Can you work these out from the model? Positions are in its coordinate system, mm. A direction names the side the tool comes from. Round coordinates to 2 decimals unless told otherwise and drop trailing zeros. Loops run counter-clockwise (first coordinate to the right, second up) from the corner with the lowest first, then second, coordinate; pieces in that order, holes last. Notation, with made-up numbers: (40, 41.5) -> (66, 41.5) arc R32 cw to (66, 76.5) -> close; hole circle Ø4 at (75.25, 85.25). An arc over 180 degrees is marked (long way). Use a Markdown table: item, result.
from build123d import *

# Parameters (mm, degrees)
SALIENTE_EXTRUIR1_DEPTH = 28
VACIADO2_START          = 6
VACIADO2_OUTLINE_W      = 16
VACIADO2_OUTLINE_H      = 23
VACIADO2_DEPTH          = 21
CORTAR_EXTRUIR1_REACH   = 46.204
CROQUIS2_W              = 6.4
CROQUIS2_H              = 10
CORTAR_EXTRUIR2_REACH   = 46.204
CROQUIS4_W              = 6.4
CROQUIS4_H              = 10


# Read off the part's stored shape, not the designer's step: Vaciado2
with BuildPart() as part:
    # Croquis1 → Saliente-Extruir1 (new body)
    with BuildSketch(Plane(origin=(0, 0, 0), x_dir=(0, 0, -1), z_dir=(1, 0, 0))):
        Polygon((0, 0), (27, 0), (27, 27), (21, 27), (0, 6), align=None)
    extrude(amount=SALIENTE_EXTRUIR1_DEPTH)

    # Vaciado2 outline → Vaciado2 (cut)
    with BuildSketch(Plane(origin=(0, 0, 0), x_dir=(1, 0, 0), z_dir=(0, 1, 0)).offset(VACIADO2_START)):
        with Locations((14, 9.5)):
            Rectangle(VACIADO2_OUTLINE_W, VACIADO2_OUTLINE_H)
    extrude(amount=VACIADO2_DEPTH, mode=Mode.SUBTRACT)

    # Croquis2 → Cortar-Extruir1 (cut, up to next)
    with BuildSketch(Plane.XY.offset(-21), mode=Mode.PRIVATE) as cortar_extruir1_sk1:
        with Locations((14, 15)):
            Rectangle(CROQUIS2_W, CROQUIS2_H)
    cortar_extruir1_tool1 = extrude(cortar_extruir1_sk1.sketch, amount=-CORTAR_EXTRUIR1_REACH, mode=Mode.PRIVATE) & part.part
    add(cortar_extruir1_tool1.solids().sort_by_distance((14, 15, -21))[0], mode=Mode.SUBTRACT)

    # Croquis4 → Cortar-Extruir2 (cut, up to next)
    with BuildSketch(Plane(origin=(0, 6, 0), x_dir=(1, 0, 0), z_dir=(0, 1, 0)), mode=Mode.PRIVATE) as cortar_extruir2_sk1:
        with Locations((14, 12)):
            Rectangle(CROQUIS4_W, CROQUIS4_H)
    cortar_extruir2_tool1 = extrude(cortar_extruir2_sk1.sketch, amount=-CORTAR_EXTRUIR2_REACH, mode=Mode.PRIVATE) & part.part
    add(cortar_extruir2_tool1.solids().sort_by_distance((14, 6, -12))[0], mode=Mode.SUBTRACT)


solid = part.part
1. Which directions (+Z, -Z, +X, -X, +Y, -Y) give clear straight access to the entire face, cutting with the end or side of a thin tool? Please do faces 1 (the flat face through (10, 6, -11)), 2 (the flat face through (17.2, 3, -12)), 3 (the flat face through (14, 10, -24)).
Answer sheet:
| item | result |
|---|---|
| face 1 | +Z, +Y |
| face 2 | +Y, -Y |
| face 3 | +Z, -Z |
2. If we mould it in two halves opening along Z, with no side actions, what happens to faces 4 (the flat face through (14, 3, 0)), 5 (the flat face through (22, 12, -15)), 6 (the flat face through (14, 3, -7))? For each: +Z half, -Z half, draft (parallel to the pull), parting line (faces both ways), or undercut.
Answer sheet:
| item | result |
|---|---|
| face 4 | +Z half |
| face 5 | draft |
| face 6 | undercut |
3. I want a section at C-C (z = -24). Please give me the cut outline in (x, y).
Answer sheet:
| item | result |
|---|---|
| outline | (0, 0) -> (28, 0) -> (28, 27) -> (0, 27) -> close; hole (10.8, 10) -> (17.2, 10) -> (17.2, 20) -> (10.8, 20) -> close |
4. I want a section at D-D (y = 5.5). Please give me the cut outline in (x, z).
Answer sheet:
| item | result |
|---|---|
| outline | (0, -27) -> (28, -27) -> (28, 0) -> (0, 0) -> close; hole (10.8, -17) -> (17.2, -17) -> (17.2, -7) -> (10.8, -7) -> close |
5. Will these pins go through, and if not, where does the flat tip stop? pin 1 Ø1 at (y, z) = (15.5, -8) entering from -X; pin 2 Ø12 at (x, z) = (22, -9.5) entering from +Y; pin 3 Ø8 at (x, z) = (9.5, -14) entering from +Y; pin 4 Ø1.5 at (x, y) = (9, 10) entering from +Z.
Answer sheet:
| item | result |
|---|---|
| pin 1 | passes through |
| pin 2 | stops at y = 21.5 |
| pin 3 | stops at y = 21.94 |
| pin 4 | stops at z = -21 |
6. I want a section at B-B (x = 16). Please give me the cut outline in (y, z).
Answer sheet:
| item | result |
|---|---|
| outline | (0, -27) -> (10, -27) -> (10, -21) -> (6, -21) -> (6, -17) -> (0, -17) -> close; (0, -7) -> (6, -7) -> (6, 0) -> (0, 0) -> close; (20, -27) -> (27, -27) -> (27, -21) -> (20, -21) -> close |
7. I want a section at A-A (y = 19.25). Please give me the cut outline in (x, z), plus the area to 3 significant figures.
Answer sheet:
| item | result |
|---|---|
| outline | (0, -27) -> (10.8, -27) -> (10.8, -21) -> (6, -21) -> (6, -13.25) -> (0, -13.25) -> close; (17.2, -27) -> (28, -27) -> (28, -13.25) -> (22, -13.25) -> (22, -21) -> (17.2, -21) -> close |
| area | 223 mm² |
8. I need wall thicknesses on line 1 (X direction, y = 11, z = -16.75); line 2 (Z direction, x = 16, y = 5.25); line 3 (Y direction, x = 13, z = -25.25). Which ranges of each line are inside material? Lowest first, please.
Answer sheet:
| item | result |
|---|---|
| line 1 | x = 0 to 6, 22 to 28 |
| line 2 | z = -27 to -17, -7 to 0 |
| line 3 | y = 0 to 10, 20 to 27 |
